Autodesk Inventor part; units mm, degrees
ref_plane "YZ Plane" through (0, 0, 0) normal (1, 0, 0) x (0, 1, 0)
ref_plane "XZ Plane" through (0, 0, 0) normal (0, 1, 0) x (-1, 0, 0)
ref_plane "XY Plane" through (0, 0, 0) normal (0, 0, 1) x (1, 0, 0)
sketch "Sketch4" plane through (0, 0, 0) normal (0, 1, 0) x (-1, 0, 0)
  line L0 (0, 0) -> (0, 66)
  line L1 (0, 66) -> (15, 66)
  line L2 (15, 66) -> (15, 50.5)
  line L3 (15, 50.5) -> (5, 50.5)
  line L4 (5, 50.5) -> (5, 46.5)
  line L5 (5, 46.5) -> (15, 46.5)
  line L6 (15, 46.5) -> (15, 0)
  line L7 (15, 0) -> (0, 0)
  dimension "d6" = 66
  dimension "d7" = 15
  dimension "d8" = 15.5
  dimension "d9" = 10
  dimension "d10" = 4
revolve "Revolution1" add sketch "Sketch4" angle 360 about axis through (-15, 0, 0) along (1, 0, 0)
sketch "Sketch5" plane through (-15, 0, 0) normal (-1, 0, 0) x (0, 0, 1)
  point P0 (0, 0)
sketch "Sketch6" plane through (-15, 0, 0) normal (-1, 0, 0) x (0, 0, 1)
  circle A0 centre (0, 0) radius 59
  point P0 (59, 0)
  point P1 (0, -59)
  point P2 (-59, 0)
  point P3 (0, 59)
  dimension "d13" = 118
hole "Hole1" at (-15, 0, 59) at (-15, -59, 0) at (-15, 0, -59) at (-15, 59, 0) direction (1, 0, 0) diameter 6.6 end through all
sketch "Sketch7" plane through (-15, 0, 0) normal (-1, 0, 0) x (0, 0, 1)
  circle A0 centre (0, 0) radius 31.5
  point P0 (31.5, 0)
  dimension "d21" = 63
hole "Hole2" at (-15, 0, 31.5) direction (1, 0, 0) diameter 6.6 end through all
sketch "Sketch8" plane through (-15, 0, 0) normal (-1, 0, 0) x (0, 0, 1)
  circle A0 centre (0, 0) radius 31.5
  point P0 (-31.5, 0)
  dimension "d29" = 63
hole "Hole3" at (-15, 0, -31.5) direction (1, 0, 0) diameter 13.835 end through all
properties part number "100mm-FlangeBottom-Sketch"
Can you work these out from the model? Positions are in its coordinate system, mm. A direction names the side the tool comes from. Round coordinates to 2 decimals unless told otherwise and drop trailing zeros. Write each loop counter-clockwise with the first axis right and the second up, starting at its lowest first coordinate (ties: lowest second). Pieces come first, ordered by that corner, then holes. Notation, with made-up numbers: (-12.75, -18) -> (6.25, -18) arc R16 cw to (6.25, -10) -> close; hole circle Ø7 at (13, 20.25). An arc over 180 degrees is marked (long way). One line per question, with ' | ' between items. Start each with the question number.
1) Suppose I cut it at A-A on x = -10.75. Count the separate pieces of the cut face and the enclosed holes in it, then the cut area to 3 significant figures.
2) Suppose I cut it at C-C on z = 0. Write out the boundary of the cut face in (x, y), then the cut area to 3 significant figures.
3) If we mould it in two halves opening along Z, with no side actions, what happens to faces 3 (the cylindrical face through (-9.93, 49.3, -10.95)), 4 (the cylindrical face through (-7.605, -25.278, 60.967)), 5 (the flat face through (0, -1, -1))? For each: released by +Z, released by -Z, zero draft, split by the parting line, or undercut.
4) Suppose I cut it at D-D on x = -2.5. Write out the boundary of the cut face in (y, z) (1 decimal), then the cut area to 3 significant figures.
5) I need wall thicknesses on line 1 (Z direction, x = -4, y = 0); line 2 (Y direction, x = -13.75, z = -32.5); line 3 (Y direction, x = -10.5, z = 36.5). Which ranges of each line are inside material? Lowest first, please. Write a range as [from, to].
6) I'm going to push flat-ended pins straight in: P1, Ø10.5, axis at y = 0, z = 59, coming from the -X side; P2, Ø5, axis at x = -5, y = 32, coming from the -Z side; P3, Ø1, axis at x = -11, y = 49.5, coming from the -Z side; P4, Ø8, axis at x = -12.5, y = -33, coming from the +Z side. Where does each tip first touch, or does it pass through?
7) On a 3-axis mill with a long thin cutter (end or side, diameter ignored), from which of +Z, -Z, +X, -X, +Y, -Y can I reach the whole of each face in a straight line? I mean faces 1 (the cylindrical face through (-7.4, -0.1, -62.3)), 2 (the cylindrical face through (-10.07, 13.97, 44.35)). Say none if no direction works.
8) Suppose I cut it at B-B on y = 0. Write out the boundary of the cut face in (x, z).
Return value:
1) separate pieces: 2 | enclosed holes: 7 | area: 12,100 mm2
2) outline: (-15, -66) -> (0, -66) -> (0, -62.3) -> (-15, -62.3) -> close; (-15, -55.7) -> (0, -55.7) -> (0, 55.7) -> (-15, 55.7) -> (-15, 50.5) -> (-5, 50.5) -> (-5, 46.5) -> (-15, 46.5) -> (-15, -46.5) -> (-5, -46.5) -> (-5, -50.5) -> (-15, -50.5) -> close; (-15, 62.3) -> (0, 62.3) -> (0, 66) -> (-15, 66) -> close | area: 1,700 mm2
3) face 3: undercut | face 4: split by the parting line | face 5: zero draft
4) outline: circle Ø132 at (0, 0); hole circle Ø6.6 at (-59, 0); hole circle Ø13.8 at (0, -31.5); hole circle Ø6.6 at (0, -59); hole circle Ø6.6 at (0, 31.5); hole circle Ø6.6 at (0, 59); hole circle Ø6.6 at (59, 0) | area: 13,400 mm2
5) line 1: z = [-66, -62.3], [-55.7, -38.42], [-24.58, 28.2], [34.8, 55.7], [62.3, 66] | line 2: y = [-57.44, -38.65], [-33.26, -6.84], [6.84, 33.26], [38.65, 57.44] | line 3: y = [-54.99, -34.9], [-28.81, 28.81], [34.9, 54.99]
6) P1: stops at x = -15 | P2: stops at z = -59.04 | P3: stops at z = -44.22 | P4: stops at z = 59.29
7) face 1: +X, -X | face 2: -X
8) outline: (-15, -66) -> (0, -66) -> (0, -62.3) -> (-15, -62.3) -> close; (-15, -55.7) -> (0, -55.7) -> (0, -38.42) -> (-15, -38.42) -> (-15, -46.5) -> (-5, -46.5) -> (-5, -50.5) -> (-15, -50.5) -> close; (-15, -24.58) -> (0, -24.58) -> (0, 28.2) -> (-15, 28.2) -> close; (-15, 34.8) -> (0, 34.8) -> (0, 55.7) -> (-15, 55.7) -> (-15, 50.5) -> (-5, 50.5) -> (-5, 46.5) -> (-15, 46.5) -> close; (-15, 62.3) -> (0, 62.3) -> (0, 66) -> (-15, 66) -> close
